Input: part model. Units: mm. Frame: model coordinates. Give positions to 0.01 mm unless a question says otherwise; leave off trailing zeros. Loops run counter-clockwise (first coordinate to the right, second up) from the corner with the lowest first, then second, coordinate; pieces in that order, holes last.
from build123d import *

# Parameters (mm, degrees)
F0_W     = 25
F0_H     = 25
F1_DEPTH = 25
F3_D     = 3
F5_D     = 3


with BuildPart() as f1:
    # F0 (on Top) → F1 (new body)
    with BuildSketch(Plane.XY):
        Rectangle(F0_W, F0_H)
    extrude(amount=F1_DEPTH)

    # F3 (through all)
    with Locations(Plane.XY.offset(25)):
        with Locations((-6, -6)):
            Hole(F3_D / 2)

    # F5 (through all)
    with Locations(Plane.XY.offset(25)):
        with Locations((4, 4)):
            Hole(F5_D / 2)


solid = f1.part
(1) Cut plane C-C (z = 7). Return the cut outline in (x, y), and give its area (3 significant figures).
Values follow:
outline: (-12.5, -12.5) - (12.5, -12.5) - (12.5, 12.5) - (-12.5, 12.5) - close; hole circle Ø3 at (-6, -6); hole circle Ø3 at (4, 4)
area: 611 mm2
(2) Cut plane B-B (y = 4). Return the cut outline in (x, z), and give its area (3 significant figures).
Values follow:
outline: (-12.5, 0) - (2.5, 0) - (2.5, 25) - (-12.5, 25) - close; (5.5, 0) - (12.5, 0) - (12.5, 25) - (5.5, 25) - close
area: 550 mm2
(3) Ray query, probe 1 along Y at (x, z) = (-6, 5.75); probe 2 along Y at (x, z) = (4, 12.25); probe 3 along X at (y, z) = (3, 22). Return the intervals inside material, ascending.
Values follow:
probe 1: y = -12.5 to -7.5, -4.5 to 12.5
probe 2: y = -12.5 to 2.5, 5.5 to 12.5
probe 3: x = -12.5 to 2.88, 5.12 to 12.5
(4) Cut plane A-A (x = -6). Return the cut outline in (y, z).
Values follow:
outline: (-12.5, 0) - (-7.5, 0) - (-7.5, 25) - (-12.5, 25) - close; (-4.5, 0) - (12.5, 0) - (12.5, 25) - (-4.5, 25) - close
(5) Mould query, pull axis X, two halves, no side actions, for faces 1 (the flat face through (-12.5, 0, 12)), 2 (the flat face through (0, -12.5, 12)), 3 (the cylindrical face through (2.57, 4.45, 12.33)), 4 (the cylindrical face through (-4.8, -6.9, 12.3)). Classes: +X half, -X half, draft (parallel to the pull), parting line (faces both ways), or undercut.
Values follow:
face 1: -X half
face 2: draft
face 3: undercut
face 4: undercut
(6) Pin query (flat end, axial travel): pin 1 Ø4 at (x, y) = (-7, -1) entering from -Z. Return the tip coordinate at first contact, or that it passes through.
Values follow:
pin 1: stops at z = 0
